```python
from build123d import *

# Parameters (mm, degrees)
ESQUISSE1_W        = 330
ESQUISSE1_H        = 330
ESQUISSE1_W_2      = 250
ESQUISSE1_H_2      = 250
BOSS_EXTRU_1_DEPTH = 200


with BuildPart() as part:
    # Esquisse1 → Boss.-Extru.1 (new body)
    with BuildSketch(Plane(origin=(0, 0, 0), x_dir=(1, 0, 0), z_dir=(0, 1, 0))):
        Rectangle(ESQUISSE1_W, ESQUISSE1_H)
        Rectangle(ESQUISSE1_W_2, ESQUISSE1_H_2, mode=Mode.SUBTRACT)
    extrude(amount=-BOSS_EXTRU_1_DEPTH)


solid = part.part
```
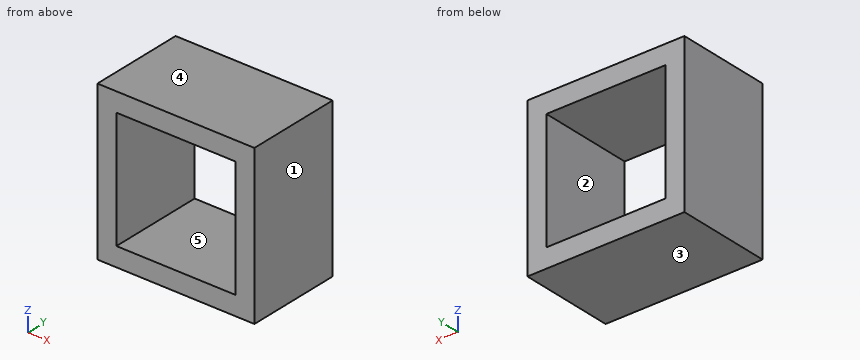
Geometry: final body of the model. Coordinates: model frame, mm. Face numbers are marked on the shaded views. A direction names the side the tool comes from. Round coordinates to 2 decimals unless told otherwise and drop trailing zeros. Loops run counter-clockwise (first coordinate to the right, second up) from the corner with the lowest first, then second, coordinate; pieces in that order, holes last. Notation, with made-up numbers: (7.5, -23.75) -> (45.5, -23.75) arc R36 cw to (45.5, 10.25) -> close; hole circle Ø1 at (39, 21.25). An arc over 180 degrees is marked (long way). Write each question's results on one line, items separated by ' | '.
Item 1: Cut plane B-B on x = -81.5. Return the cut outline in (y, z).
Answers below:
outline: (-200, -165) -> (0, -165) -> (0, -125) -> (-200, -125) -> close; (-200, 125) -> (0, 125) -> (0, 165) -> (-200, 165) -> close
Item 2: Cut plane A-A on z = -104.5. Return the cut outline in (x, y), and give its area (3 significant figures).
Answers below:
outline: (-165, -200) -> (-125, -200) -> (-125, 0) -> (-165, 0) -> close; (125, -200) -> (165, -200) -> (165, 0) -> (125, 0) -> close | area: 16,000 mm²
Item 3: Pull-direction query (Z, two-part tool) for the marked faces 1, 2 and 3; classes: pulls with the +Z half, pulls with the -Z half, needs draft (parallel to the pull), parting line crosses it, or undercut.
Answers below:
face 1: needs draft | face 2: undercut | face 3: pulls with the -Z half
Item 4: Cut plane C-C on y = -48.5. Return the cut outline in (x, z).
Answers below:
outline: (-165, -165) -> (165, -165) -> (165, 165) -> (-165, 165) -> close; hole (-125, -125) -> (125, -125) -> (125, 125) -> (-125, 125) -> close
Item 5: Set-up query: the marked faces 4 and 5. Return all of +Z, -Z, +X, -X, +Y, -Y with unobstructed straight access to the full face (end or side cutting, diameter ignored); none if empty.
Answers below:
face 4: +Z, +X, -X, +Y, -Y | face 5: +Y, -Y
Item 6: Pin query (flat end, axial travel): pin 1 Ø10 at (x, z) = (95.5, 123.5) entering from +Y. Return the tip coordinate at first contact, or that it passes through.
Answers below:
pin 1: stops at y = 0
Item 7: Line query: probe 1 along Z at (x, y) = (38, -174). Output: solid intervals per line, ascending. Write a range as [from, to].
Answers below:
probe 1: z = [-165, -125], [125, 165]
